Read the model definition and answer for the solid it produces. Units are mm, in the model's axes. A direction names the side the tool comes from. Give positions to 0.01 mm unless a question says otherwise; leave off trailing zeros. Write each loop counter-clockwise with the first axis right and the second up, starting at its lowest first coordinate (ties: lowest second). Pieces come first, ordered by that corner, then holes. Notation, with made-up numbers: (-15.75, -18.75) - (28.25, -18.75) arc R8 cw to (28.25, -6.75) - close; hole circle Ø8 at (-25.5, -12). An arc over 180 degrees is marked (long way). Answer as CSV lines item,"result".
```python
from build123d import *

# Parameters (mm, degrees)
F0_R     = 20.7
F0_R_2   = 17.5
F1_DEPTH = 41
F0_R_3   = 14.5
F2_DEPTH = 3
F4_R     = 17.5
F4_R_2   = 12.5
F4_R_3   = 4
F6_DEPTH = 4
F7_DEPTH = 25
F9_DEPTH = 21.5


with BuildPart() as f1:
    # F0 (on Top) → F1 (new body)
    with BuildSketch(Plane.XY):
        Circle(F0_R)
        Circle(F0_R_2, mode=Mode.SUBTRACT)
    extrude(amount=F1_DEPTH)

    # F0 (on Top) → F2 (join)
    with BuildSketch(Plane.XY):
        Circle(F0_R_2)
        Circle(F0_R_3, mode=Mode.SUBTRACT)
    extrude(amount=F2_DEPTH)

    # F4 (on offset) → F5 (join, up to the next surface of F1)
    with BuildSketch(Plane.XZ.offset(25.5)):
        with Locations((0, 20.5)):
            Circle(F4_R)
        with Locations((0, 20.5)):
            Circle(F4_R_2, mode=Mode.SUBTRACT)
        with Locations((0, 20.5)):
            Circle(F4_R_2)
        with Locations((0, 20.5)):
            Circle(F4_R_3, mode=Mode.SUBTRACT)
    extrude(until=Until.NEXT, dir=(0, 1, 0))

    # F4 (on offset) → F6 (cut)
    with BuildSketch(Plane.XZ.offset(25.5)):
        with Locations((0, 20.5)):
            Circle(F4_R)
        with Locations((0, 20.5)):
            Circle(F4_R_2, mode=Mode.SUBTRACT)
    extrude(amount=-F6_DEPTH, mode=Mode.SUBTRACT)

    # F4 (on offset) → F7 (cut)
    with BuildSketch(Plane.XZ.offset(25.5)):
        with Locations((0, 20.5)):
            Circle(F4_R_3)
    extrude(amount=-F7_DEPTH, mode=Mode.SUBTRACT)

    # F8 (on Front) → F9 (cut, through all)
    with BuildSketch(Plane.XZ):
        Polygon((5.15, 23.43514415), (0, 26.4084980363), (-5.15, 23.43514415), (-5.15, 17.4884363773), (0, 14.515082491), (5.15, 17.4884363773), align=None)
    extrude(amount=F9_DEPTH, mode=Mode.SUBTRACT)


solid = f1.part
```
(1) A cutting plane is placed at D-D (y = -12.5). Write down the section's boundary in (x, z).
Worked out:
outline,"(-16.5, 0) - (-7.35, 0) - (-7.35, 3) - (-12.25, 3) - (-12.25, 41) - (-16.5, 41) - (-16.5, 26.33) arc R17.5 ccw to (-16.5, 14.67) - close; (7.35, 0) - (16.5, 0) - (16.5, 14.67) arc R17.5 ccw to (16.5, 26.33) - (16.5, 41) - (12.25, 41) - (12.25, 3) - (7.35, 3) - close"
(2) A cutting plane is placed at B-B (x = 7). Write down the section's boundary in (y, z), and give its area (3 significant figures).
Worked out:
outline,"(-25.5, 10.14) - (-21.5, 10.14) - (-21.5, 4.46) - (-19.48, 4.46) - (-19.48, 0) - (-12.7, 0) - (-12.7, 3) - (-16.04, 3) - (-16.04, 41) - (-19.48, 41) - (-19.48, 36.54) - (-21.5, 36.54) - (-21.5, 30.86) - (-25.5, 30.86) - close; (12.7, 0) - (19.48, 0) - (19.48, 41) - (16.04, 41) - (16.04, 3) - (12.7, 3) - close"
area,"450 mm^2"
(3) Find the intervals of material crossed by L1, parallel to Y at x = 0, z = 1.45; L2, parallel to Y at x = 0, z = 26; L3, parallel to Z at x = 0, y = -24.25, in increasing order.
Worked out:
L1,"y = -20.7 to -14.5, 14.5 to 20.7"
L2,"y = -25.5 to -21.5, 17.5 to 20.7"
L3,"z = 8 to 16.5, 24.5 to 33"
(4) A cutting plane is placed at C-C (z = 9.5). Write down the section's boundary in (x, y).
Worked out:
outline,"(-13.61, -21.5) - (-5.94, -21.5) - (-5.94, -25.5) - (5.94, -25.5) - (5.94, -21.5) - (13.61, -21.5) - (13.61, -15.6) arc R20.7 ccw (long way) to (-13.61, -15.6) - close; hole circle Ø35 at (0, 0)"
(5) A cutting plane is placed at A-A (y = 0). Write down the section's boundary in (x, z), and give its area (3 significant figures).
Worked out:
outline,"(-20.7, 0) - (-14.5, 0) - (-14.5, 3) - (-17.5, 3) - (-17.5, 41) - (-20.7, 41) - close; (14.5, 0) - (20.7, 0) - (20.7, 41) - (17.5, 41) - (17.5, 3) - (14.5, 3) - close"
area,"280 mm^2"
(6) For faces 1 (the cylindrical face through (-12.898, -17.512, 32.327)), 2 (the flat face through (-2.54, -19.08, 24.94)), 3 (the flat face through (-7, 13, 3)), 4 (the flat face through (4.3, 14.1, 0)), determine the directions among +Z, -Z, +X, -X, +Y, -Y from which every point of the face is accessible in a straight line to the end or side of a thin tool.
Worked out:
face 1,"-Y"
face 2,"none"
face 3,"+Z"
face 4,"-Z, +X, -X, +Y, -Y"
(7) Each of these flat-tipped pins is pushed along its axis until it touches: P1, Ø10, axis at x = 15.5, z = 4.5, coming from the +Y side; P2, Ø5, axis at x = -11, z = 36, coming from the +Y side; P3, Ø3, axis at x = -1.5, z = 22, coming from the +Y side; P4, Ø3, axis at x = -5, y = 13.5, coming from the -Z side. Where does it stop, or does it pass through?
Worked out:
P1,"stops at y = 17.84"
P2,"stops at y = 18.87"
P3,"stops at y = 20.7"
P4,"stops at z = 0"
(8) The mould has two halves that part along Z. Classify faces 5 (the cylindrical face through (-0.521, -23.528, 24.466)), 6 (the cylindrical face through (6.691, -12.864, 1.479)), 7 (the flat face through (-5, 17, 41)): +Z half, -Z half, draft (parallel to the pull), parting line (faces both ways), or undercut.
Worked out:
face 5,"undercut"
face 6,"draft"
face 7,"+Z half"
